from build123d import *

# Parameters (mm, degrees)
SKETCH2_W           = 96
SKETCH2_H           = 64
BOSS_EXTRUDE1_DEPTH = 16
CUT_EXTRUDE1_DEPTH  = 16
BOSS_EXTRUDE2_DEPTH = 16
SKETCH11_W          = 24
SKETCH11_H          = 42
BOSS_EXTRUDE3_DEPTH = 28
BOSS_EXTRUDE4_DEPTH = 12
CUT_EXTRUDE2_START  = -42
SKETCH16_R          = 6
CUT_EXTRUDE2_DEPTH  = 42


with BuildPart() as part:
    # Sketch2 → Boss-Extrude1 (new body)
    with BuildSketch(Plane(origin=(0, 0, 0), x_dir=(1, 0, 0), z_dir=(0, 1, 0))):
        Rectangle(SKETCH2_W, SKETCH2_H)
    extrude(amount=BOSS_EXTRUDE1_DEPTH)

    # Sketch5 → Cut-Extrude1 (cut)
    with BuildSketch(Plane(origin=(0, 16, 0), x_dir=(1, 0, 0), z_dir=(0, 1, 0))):
        with BuildLine():
            Line((48, -16), (28, -16))
            ThreePointArc((28, -16), (20, -8), (28, 0))
            Line((28, 0), (48, 0))
            ThreePointArc((48, 0), (56, -8), (48, -16))
        make_face()
    extrude(amount=-CUT_EXTRUDE1_DEPTH, mode=Mode.SUBTRACT)

    # Sketch10 → Boss-Extrude2 (add)
    with BuildSketch(Plane.ZY.offset(48)):
        with BuildLine():
            Line((32, 0), (-32, 0))
            Line((-32, 0), (-32, 64))
            Line((-32, 64), (-16, 64))
            ThreePointArc((-16, 64), (17.941125497, 49.941125497), (32, 16))
            Line((32, 16), (32, 0))
        make_face()
    extrude(amount=-BOSS_EXTRUDE2_DEPTH)

    # Sketch11 → Boss-Extrude3 (add)
    with BuildSketch(Plane(origin=(0, 16, 0), x_dir=(1, 0, 0), z_dir=(0, 1, 0))):
        with Locations((-20, 11)):
            Rectangle(SKETCH11_W, SKETCH11_H)
    extrude(amount=BOSS_EXTRUDE3_DEPTH)

    # Sketch15 → Boss-Extrude4 (add)
    with BuildSketch(Plane(origin=(0, 0, -32), x_dir=(-1, 0, 0), z_dir=(0, 0, -1))):
        Polygon((-48, 16), (8, 44), (8, 16), align=None)
    extrude(amount=-BOSS_EXTRUDE4_DEPTH)

    # Sketch16 → Cut-Extrude2 (cut)
    with BuildSketch(Plane(origin=(0, 0, -32), x_dir=(-1, 0, 0), z_dir=(0, 0, -1)).offset(CUT_EXTRUDE2_START)):
        with Locations((20, 44)):
            Circle(SKETCH16_R)
    extrude(amount=CUT_EXTRUDE2_DEPTH, mode=Mode.SUBTRACT)


solid = part.part
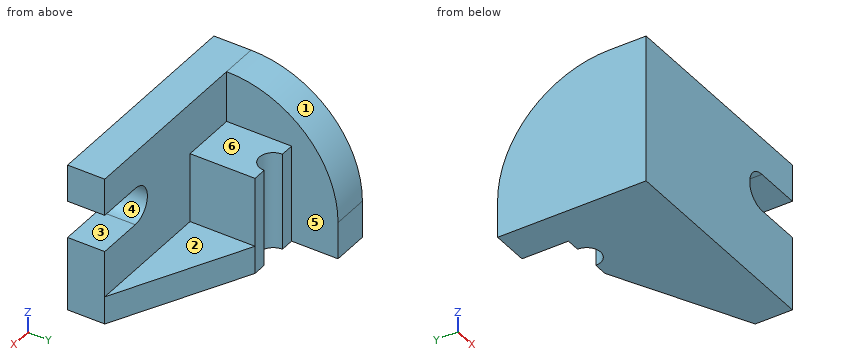
Work out the finished part from the listing and answer in its coordinate system (mm). Face numbers are marked on the shaded views. A direction names the side the tool comes from. Coordinates: 2 decimals unless noted, no trailing zeros. Write each loop counter-clockwise with the first axis right and the second up, starting at its lowest first coordinate (ties: lowest second). Pieces come first, ordered by that corner, then holes.
1. Consider line 1 along Z through (x, y) = (38.5, 14); line 2 along Y through (x, z) = (43, 21); line 3 along Y through (x, z) = (-20, -14). Determine where each line is inside the solid, lowest interval first.
Results list:
line 1: z = -32 to 0, 16 to 32
line 2: y = 0 to 16
line 3: y = 0 to 38
2. The part is cut by section C-C, the plane x = 2.5. Write down the section's boundary in (y, z), and give its area (3 significant figures).
Results list:
outline: (0, -32) - (38.75, -32) - (38.75, -20) - (16, -20) - (16, 32) - (0, 32) - close
area: 1,300 mm2
3. The part is cut by section D-D, the plane y = 57. Write down the section's boundary in (x, z).
Results list:
outline: (-48, -32) - (-32, -32) - (-32, 8.96) - (-48, 8.96) - close
4. Flat-ended cylindrical pins translate along their axes: pin 1 (4 mm diameter, centred on x = -35, y = 46, fed in from +Z); pin 2 (8.5 mm diameter, centred on y = 30, z = 1.5, fed in from +X); pin 3 (5 mm diameter, centred on x = -17.5, y = 41.5, fed in from +Z). Find the tip coordinate at first contact, or state that the pin passes through.
Results list:
pin 1: stops at z = 22.99
pin 2: stops at x = -8
pin 3: stops at z = 10
5. For the marked faces 1, 2 and 3, determine the directions among +Z, -Z, +X, -X, +Y, -Y from which every point of the face is accessible in a straight line to the end or side of a thin tool.
Results list:
face 1: +Z, +X, -X, +Y
face 2: +Z, +X, +Y
face 3: +X, +Y, -Y
6. For a pull along Z with two mould halves and no side action, classify the marked faces 4, 5 and 6 as +Z half, -Z half, draft (parallel to the pull), parting line (faces both ways), or undercut.
Results list:
face 4: undercut
face 5: draft
face 6: +Z half
7. The part is cut by section B-B, the plane z = 8. Write down the section's boundary in (x, y), and give its area (3 significant figures).
Results list:
outline: (-48, 0) - (20, 0) - (20, 16) - (-8, 16) - (-8, 44) - (-14, 44) arc R6 cw to (-26, 44) - (-32, 44) - (-32, 57.57) - (-48, 57.57) - close
area: 2,370 mm2
8. The part is cut by section A-A, the plane x = 37. Write down the section's boundary in (y, z), and give its area (3 significant figures).
Results list:
outline: (0, -32) - (21.5, -32) - (21.5, -20) - (16, -20) - (16, 0) - (0, 0) - close; (0, 16) - (16, 16) - (16, 32) - (0, 32) - close
area: 834 mm2
